Source: CAD feature listing. Evaluate the final solid. Frame: model axes, mm. Face numbers are marked on the shaded views. A direction names the side the tool comes from. Coordinates: 2 decimals unless noted, no trailing zeros. Order: outer loops, then holes, each group sorted by start corner. A loop starts at its lowest first (then second) coordinate and runs counter-clockwise, first axis right, second up.
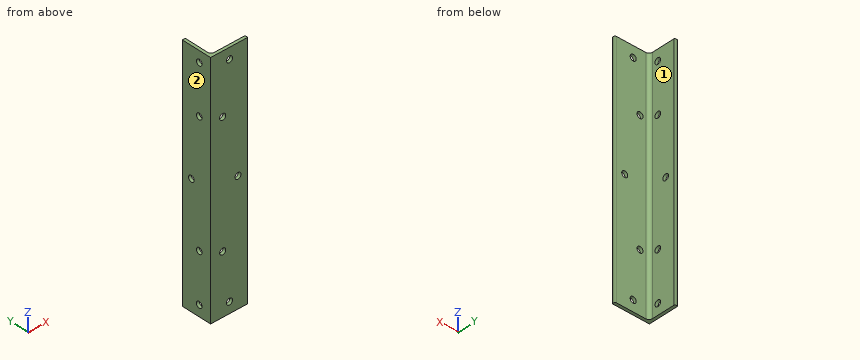
```python
from build123d import *

# Parameters (mm, degrees)
F1_DEPTH = 990
F2_R     = 14
F3_R     = 4.6
F5_D     = 25
F7_D     = 25
F9_D     = 25


with BuildPart() as f1:
    # F0 (on Top) → F1 (new body)
    with BuildSketch(Plane.XY):
        Polygon((0, 125), (0, 0), (153.050105, 0), (153.050105, 12), (12, 12), (12, 125), align=None)
    extrude(amount=F1_DEPTH)

    # F2
    f2_edges = [f1.edges().sort_by_distance(p)[0] for p in [
        (12, 12, 495),
    ]]
    fillet(f2_edges, radius=F2_R)

    # F3
    f3_edges = [f1.edges().sort_by_distance(p)[0] for p in [
        (12, 125, 495),
        (153.050105, 12, 495),
    ]]
    fillet(f3_edges, radius=F3_R)

    # F5 (through all)
    with Locations(Plane(origin=(0, 12, 0), x_dir=(-1, 0, 0), z_dir=(0, 1, 0))):
        with Locations((-113.050105, 495)):
            Hole(F5_D / 2)

    # F7 (through all)
    with Locations(Plane(origin=(0, 12, 0), x_dir=(-1, 0, 0), z_dir=(0, 1, 0))):
        with Locations((-78.050105, 945), (-50, 745), (-50, 245), (-78.050105, 45)):
            Hole(F7_D / 2)

    # F9 (through all)
    with Locations(Plane.YZ.offset(12)):
        with Locations((50, 945), (50, 745), (85, 495), (50, 245), (50, 45)):
            Hole(F9_D / 2)


solid = f1.part
```
1. Ray query, line 1 (Z direction, x = 9.25, y = 50); line 2 (Z direction, x = 50, y = 7.75); line 3 (Z direction, x = 2, y = 85). Return the intervals inside material, ascending.
Findings:
line 1: z = 0 to 32.5, 57.5 to 232.5, 257.5 to 732.5, 757.5 to 932.5, 957.5 to 990
line 2: z = 0 to 232.5, 257.5 to 732.5, 757.5 to 990
line 3: z = 0 to 482.5, 507.5 to 990
2. Section query A-A on y = 50. Return loops of the section in (x, z), plus the area to 3 significant figures.
Findings:
outline: (0, 0) - (12, 0) - (12, 32.5) - (0, 32.5) - close; (0, 57.5) - (12, 57.5) - (12, 232.5) - (0, 232.5) - close; (0, 257.5) - (12, 257.5) - (12, 732.5) - (0, 732.5) - close; (0, 757.5) - (12, 757.5) - (12, 932.5) - (0, 932.5) - close; (0, 957.5) - (12, 957.5) - (12, 990) - (0, 990) - close
area: 10,700 mm2
3. Section query B-B on z = 745. Return loops of the section in (x, y), plus the area to 3 significant figures.
Findings:
outline: (0, 0) - (37.5, 0) - (37.5, 12) - (26, 12) arc R14 cw to (12, 26) - (12, 37.5) - (0, 37.5) - close; (0, 62.5) - (12, 62.5) - (12, 120.4) arc R4.6 ccw to (7.4, 125) - (0, 125) - close; (62.5, 0) - (153.05, 0) - (153.05, 7.4) arc R4.6 ccw to (148.45, 12) - (62.5, 12) - close
area: 2,630 mm2
4. Pin query (flat end, axial travel): P1, Ø6, axis at y = 96.5, z = 702, coming from the +X side; P2, Ø6, axis at x = 48, z = 402.5, coming from the +Y side; P3, Ø15, axis at y = 50, z = 945, coming from the +X side. Return the tip coordinate at first contact, or that it passes through.
Findings:
P1: stops at x = 12
P2: stops at y = 12
P3: passes through
5. Access query for the marked faces 1 and 2. Directions: +Z, -Z, +X, -X, +Y, -Y. A direction counts if a zero-diameter tool reaches every point of the face in a straight line with its end or side. Return the directions, or none.
Findings:
face 1: +Z, -Z, +X, +Y
face 2: +Z, -Z, -X, +Y, -Y
6. Section query D-D on z = 602. Return loops of the section in (x, y).
Findings:
outline: (0, 0) - (153.05, 0) - (153.05, 7.4) arc R4.6 ccw to (148.45, 12) - (26, 12) arc R14 cw to (12, 26) - (12, 120.4) arc R4.6 ccw to (7.4, 125) - (0, 125) - close
7. Section query C-C on x = 49.5. Return loops of the section in (y, z).
Findings:
outline: (0, 0) - (12, 0) - (12, 232.51) - (0, 232.51) - close; (0, 257.49) - (12, 257.49) - (12, 732.51) - (0, 732.51) - close; (0, 757.49) - (12, 757.49) - (12, 990) - (0, 990) - close
